from build123d import *

# Parameters (mm, degrees)
SKETCH1_R           = 31.0896
BOSS_EXTRUDE1_DEPTH = 16.002
BOSS_EXTRUDE2_START = -6.35
BOSS_EXTRUDE2_DEPTH = 6.35
FILLET2_R           = 6.35
CUT_EXTRUDE2_REACH  = 96.198
SKETCH4_R           = 1.778
SKETCH4_R_2         = 6.35
SKETCH7_R           = 2.0193
CUT_EXTRUDE4_DEPTH  = 95.197625109
FILLET7_R           = 6.35
FILLET8_R           = 41.148
CUT_EXTRUDE5_DEPTH  = 12.7
FILLET9_R           = 2.54
SKETCH9_R           = 6.35
CUT_EXTRUDE6_DEPTH  = 3.302


# Some blends are built 0.0001 mm under size
with BuildPart() as part:
    # Sketch1 → Boss-Extrude1 (new body)
    with BuildSketch(Plane(origin=(0, 0, 0), x_dir=(1, 0, 0), z_dir=(0, 1, 0))):
        with Locations(Location((0, 0, 0), (0, 0, 270))):
            Circle(SKETCH1_R)
    extrude(amount=BOSS_EXTRUDE1_DEPTH)

    # Sketch2 → Boss-Extrude2 (add)
    with BuildSketch(Plane(origin=(0, 16.002, 0), x_dir=(1, 0, 0), z_dir=(0, 1, 0)).offset(BOSS_EXTRUDE2_START)):
        with BuildLine():
            Line((-31.0896, 0), (-31.0896, 41.148))
            Line((-31.0896, 41.148), (83.2104, 41.148))
            Line((83.2104, 41.148), (83.2104, 15.748))
            Line((83.2104, 15.748), (31.0896, 15.748))
            Line((31.0896, 15.748), (31.0896, 0))
            ThreePointArc((31.0896, 0), (0, -31.0896), (-31.0896, 0))
        make_face()
    extrude(amount=BOSS_EXTRUDE2_DEPTH)

    # Fillet2
    fillet2_edges = [part.edges().sort_by_distance(p)[0] for p in [
        (31.0896, 12.827, -15.748),
    ]]
    fillet(fillet2_edges, radius=FILLET2_R)

    # Sketch4 → Cut-Extrude2 (cut, up to next)
    with BuildSketch(Plane(origin=(0, 16.002, 0), x_dir=(1, 0, 0), z_dir=(0, 1, 0)), mode=Mode.PRIVATE) as cut_extrude2_sk1:
        with Locations(Location((61.411202787, 35.362797213, 0), (0, 0, 270))):
            Circle(SKETCH4_R)
    cut_extrude2_tool1 = extrude(cut_extrude2_sk1.sketch, amount=-CUT_EXTRUDE2_REACH, mode=Mode.PRIVATE) & part.part
    # Sketch4 → Cut-Extrude2 (cut, up to next)
    with BuildSketch(Plane(origin=(0, 16.002, 0), x_dir=(1, 0, 0), z_dir=(0, 1, 0)), mode=Mode.PRIVATE) as cut_extrude2_sk2:
        with Locations(Location((75.240797213, 35.362797213, 0), (0, 0, 270))):
            Circle(SKETCH4_R)
    cut_extrude2_tool2 = extrude(cut_extrude2_sk2.sketch, amount=-CUT_EXTRUDE2_REACH, mode=Mode.PRIVATE) & part.part
    # Sketch4 → Cut-Extrude2 (cut, up to next)
    with BuildSketch(Plane(origin=(0, 16.002, 0), x_dir=(1, 0, 0), z_dir=(0, 1, 0)), mode=Mode.PRIVATE) as cut_extrude2_sk3:
        with Locations(Location((75.240797213, 21.533202787, 0), (0, 0, 270))):
            Circle(SKETCH4_R)
    cut_extrude2_tool3 = extrude(cut_extrude2_sk3.sketch, amount=-CUT_EXTRUDE2_REACH, mode=Mode.PRIVATE) & part.part
    # Sketch4 → Cut-Extrude2 (cut, up to next)
    with BuildSketch(Plane(origin=(0, 16.002, 0), x_dir=(1, 0, 0), z_dir=(0, 1, 0)), mode=Mode.PRIVATE) as cut_extrude2_sk4:
        with Locations(Location((68.326, 28.448, 0), (0, 0, 270))):
            Circle(SKETCH4_R_2)
    cut_extrude2_tool4 = extrude(cut_extrude2_sk4.sketch, amount=-CUT_EXTRUDE2_REACH, mode=Mode.PRIVATE) & part.part
    # Sketch4 → Cut-Extrude2 (cut, up to next)
    with BuildSketch(Plane(origin=(0, 16.002, 0), x_dir=(1, 0, 0), z_dir=(0, 1, 0)), mode=Mode.PRIVATE) as cut_extrude2_sk5:
        with Locations(Location((61.411202787, 21.533202787, 0), (0, 0, 270))):
            Circle(SKETCH4_R)
    cut_extrude2_tool5 = extrude(cut_extrude2_sk5.sketch, amount=-CUT_EXTRUDE2_REACH, mode=Mode.PRIVATE) & part.part
    add(cut_extrude2_tool1.solids().sort_by_distance((61.411203, 16.002, -35.362797))[0], mode=Mode.SUBTRACT)
    add(cut_extrude2_tool2.solids().sort_by_distance((75.240797, 16.002, -35.362797))[0], mode=Mode.SUBTRACT)
    add(cut_extrude2_tool3.solids().sort_by_distance((75.240797, 16.002, -21.533203))[0], mode=Mode.SUBTRACT)
    add(cut_extrude2_tool4.solids().sort_by_distance((68.326, 16.002, -28.448))[0], mode=Mode.SUBTRACT)
    add(cut_extrude2_tool5.solids().sort_by_distance((61.411203, 16.002, -21.533203))[0], mode=Mode.SUBTRACT)

    # Sketch7 → Cut-Extrude4 (cut, through all)
    with BuildSketch(Plane(origin=(0, 0, 0), x_dir=(1, 0, 0), z_dir=(0, 1, 0))):
        with BuildLine():
            ThreePointArc((27.94, 0), (22.235278576, 16.918510179), (7.450666667, 26.928259621))
            Line((7.450666667, 26.928259621), (4.402666667, 15.912153412))
            ThreePointArc((4.402666667, 15.912153412), (13.139028249, 9.997301469), (16.51, 0))
            ThreePointArc((16.51, 0), (13.139028249, -9.997301469), (4.402666667, -15.912153412))
            Line((4.402666667, -15.912153412), (7.450666667, -26.928259621))
            ThreePointArc((7.450666667, -26.928259621), (22.235278576, -16.918510179), (27.94, 0))
        make_face()
        with BuildLine():
            Line((-15.912153412, -4.402666667), (-26.928259621, -7.450666667))
            ThreePointArc((-26.928259621, -7.450666667), (-19.756563466, -19.756563466), (-7.450666667, -26.928259621))
            Line((-7.450666667, -26.928259621), (-4.402666667, -15.912153412))
            ThreePointArc((-4.402666667, -15.912153412), (-11.674332957, -11.674332957), (-15.912153412, -4.402666667))
        make_face()
        with BuildLine():
            Line((-4.402666667, 15.912153412), (-7.450666667, 26.928259621))
            ThreePointArc((-7.450666667, 26.928259621), (-19.756563466, 19.756563466), (-26.928259621, 7.450666667))
            Line((-26.928259621, 7.450666667), (-15.912153412, 4.402666667))
            ThreePointArc((-15.912153412, 4.402666667), (-11.674332957, 11.674332957), (-4.402666667, 15.912153412))
        make_face()
        with Locations(Location((-19.05, 0, 0), (0, 0, 270))):
            Circle(SKETCH7_R)
        with Locations(Location((0, -19.05, 0), (0, 0, 270))):
            Circle(SKETCH7_R)
        with Locations(Location((0, 19.05, 0), (0, 0, 270))):
            Circle(SKETCH7_R)
    extrude(amount=CUT_EXTRUDE4_DEPTH, mode=Mode.SUBTRACT)

    # Fillet7
    # the kernel refuses this fillet: 6.35 mm, written as the material it adds along each edge
    with BuildSketch(Plane(origin=(-26.928259621, 0, -7.450666667), x_dir=(0.40702884348062, 0, -0.9134153056385845), z_dir=(0, 1, 0)), Plane(origin=(-7.450666667, 0, 26.928259621), x_dir=(-0.9134153056385848, 0, -0.40702884348061963), z_dir=(0, 1, 0))) as fillet7_piece_1:
        with BuildLine():
            CenterArc((7.365726845, -6.279391075), FILLET7_R, 81.447682412, 107.104635177)
            Line((1.086335771, -7.223715029), (0, 0))
            ThreePointArc((0, 0), (4.1550254, 0.310679271), (8.3100508, 0))
        make_face()
    extrude(amount=16.002)
    with BuildSketch(Plane(origin=(-7.450666667, 0, -26.928259621), x_dir=(0.26666666666666705, 0, 0.9637888196533972), z_dir=(0, 1, 0)), Plane(origin=(7.450666667, 0, 26.928259621), x_dir=(-0.26666666666666733, 0, -0.9637888196533971), z_dir=(0, 1, 0)), Plane(origin=(-26.928259621, 0, 7.450666667), x_dir=(0.9637888196533975, 0, -0.26666666666666644), z_dir=(0, 1, 0))) as fillet7_piece_2:
        with BuildLine():
            CenterArc((7.304942452, -6.35), FILLET7_R, 90, 107.104635177)
            ThreePointArc((1.235807879, -8.217647059), (0.310679271, -4.1550254), (0, 0))
            Line((0, 0), (7.304942452, 0))
        make_face()
    extrude(amount=16.002)
    with BuildSketch(Plane(origin=(-4.402666667, 0, -15.912153412), x_dir=(-0.916852417954672, 0, 0.39922630636103035), z_dir=(0, 1, 0)), Plane(origin=(4.402666667, 0, 15.912153412), x_dir=(0.9168524179546733, 0, -0.39922630636102746), z_dir=(0, 1, 0)), Plane(origin=(-15.912153412, 0, 4.402666667), x_dir=(0.39922630636102946, 0, 0.9168524179546725), z_dir=(0, 1, 0))) as fillet7_piece_3:
        with BuildLine():
            CenterArc((5.522661099, -6.287214109), FILLET7_R, 98.063810107, 73.872379787)
            Line((-0.76455301, -5.396462319), (0, 0))
            ThreePointArc((0, 0), (2.315954654, -0.163243317), (4.631909309, 0))
        make_face()
    extrude(amount=16.002)
    with BuildSketch(Plane(origin=(4.402666667, 0, -15.912153412), x_dir=(0.26666666666666416, 0, -0.9637888196533979), z_dir=(0, 1, 0))) as fillet7_piece_4:
        with BuildLine():
            CenterArc((5.450352912, -6.35), FILLET7_R, 90, 73.872379787)
            ThreePointArc((-0.649745119, -4.586111111), (-0.163243317, -2.315954654), (0, 0))
            Line((0, 0), (5.450352912, 0))
        make_face()
    extrude(amount=16.002)
    with BuildSketch(Plane(origin=(7.450666667, 0, -26.928259621), x_dir=(-0.2666666666666666, 0, 0.9637888196533974), z_dir=(0, 1, 0))) as fillet7_piece_5:
        with BuildLine():
            CenterArc((7.304942452, 6.35), FILLET7_R, 162.895364823, 107.104635177)
            ThreePointArc((1.235807879, 8.217647059), (0.310679271, 4.1550254), (0, 0))
            Line((0, 0), (7.304942452, 0))
        make_face()
    extrude(amount=16.002)
    with BuildSketch(Plane(origin=(-4.402666667, 0, 15.912153412), x_dir=(-0.9168524179546729, 0, -0.3992263063610288), z_dir=(0, 1, 0)), Plane(origin=(-15.912153412, 0, -4.402666667), x_dir=(0.39922630636102996, 0, -0.9168524179546723), z_dir=(0, 1, 0))) as fillet7_piece_6:
        with BuildLine():
            CenterArc((5.522661099, 6.287214109), FILLET7_R, 188.063810107, 73.872379787)
            Line((-0.76455301, 5.396462319), (0, 0))
            ThreePointArc((0, 0), (2.315954654, 0.163243317), (4.631909309, 0))
        make_face()
    extrude(amount=16.002)

    # Fillet8
    fillet8_edges = [part.edges().sort_by_distance(p)[0] for p in [
        (-31.0896, 12.827, -41.148),
    ]]
    fillet(fillet8_edges, radius=FILLET8_R - 0.0001)  # a hair under: the kernel refuses the full size

    # Sketch8 → Cut-Extrude5 (cut)
    with BuildSketch(Plane.XZ):
        with BuildLine():
            Line((-10.414, 10.414), (10.414, 10.414))
            ThreePointArc((10.414, 10.414), (20.828, 0), (10.414, -10.414))
            Line((10.414, -10.414), (-10.414, -10.414))
            Line((-10.414, -10.414), (-10.414, 10.414))
        make_face()
    extrude(amount=-CUT_EXTRUDE5_DEPTH, mode=Mode.SUBTRACT)

    # Fillet9
    # the kernel refuses this fillet: 2.54 mm, written as the material it takes off along each edge
    with BuildSketch(Plane(origin=(13.087195122, 12.7, 10.065059555), x_dir=(-0.7525451578932851, 0, 0.658540648199768), z_dir=(0, -1, 0))) as fillet9_piece_1:
        with BuildLine():
            CenterArc((7.288242174, 2.538935053), FILLET9_R, 131.188669075, 137.152126286)
            Line((5.615548928, 4.450399754), (5.448279603, 4.641546224))
            ThreePointArc((5.448279603, 4.641546224), (2.074222188, 1.688960676), (-0.1125988, 0.227678524))
            Line((-0.1125988, 0.227678524), (-0.049545453, -0.249120951))
            ThreePointArc((-0.049545453, -0.249120951), (6.014734512, -0.336617786), (7.207343199, -0.253893505))
            Line((7.207343199, -0.253893505), (7.214697651, 0))
        make_face()
    extrude(amount=30.736744128, mode=Mode.SUBTRACT)
    with BuildSketch(Plane(origin=(13.087195122, 12.7, -10.065059555), x_dir=(-0.7525451578933744, 0, -0.658540648199666), z_dir=(0, -1, 0))) as fillet9_piece_2:
        with BuildLine():
            CenterArc((7.288242174, -2.538935053), FILLET9_R, 91.659204639, 137.152126286)
            Line((5.615548928, -4.450399754), (5.448279603, -4.641546224))
            ThreePointArc((5.448279603, -4.641546224), (2.074222188, -1.688960676), (-0.1125988, -0.227678524))
            Line((-0.1125988, -0.227678524), (-0.049545453, 0.249120951))
            ThreePointArc((-0.049545453, 0.249120951), (6.014734512, 0.336617786), (7.207343199, 0.253893505))
            Line((7.207343199, 0.253893505), (7.214697651, 0))
        make_face()
    extrude(amount=30.736744128, mode=Mode.SUBTRACT)

    # Sketch9 → Cut-Extrude6 (cut)
    with BuildSketch(Plane.XZ.offset(-12.7)):
        with Locations(Location((0, 0, 0), (0, 0, 270))):
            Circle(SKETCH9_R)
    extrude(amount=-CUT_EXTRUDE6_DEPTH, mode=Mode.SUBTRACT)


solid = part.part
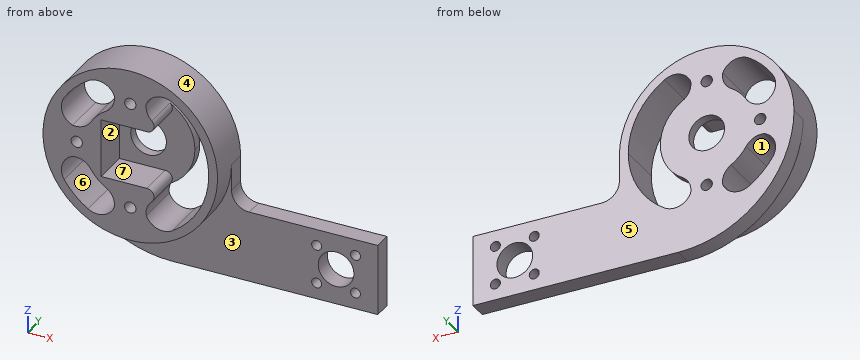
For this review, take the finished solid that the model builds, in its own axes (mm). Face numbers are marked on the shaded views. A direction names the side the tool comes from. Round coordinates to 2 decimals unless told otherwise and drop trailing zeros. Order: outer loops, then holes, each group sorted by start corner. A loop starts at its lowest first (then second) coordinate and runs counter-clockwise, first axis right, second up. Notation, with made-up numbers: M 0,19 L 23,19 A32 cw 23,47 Z; hole C -12.75,15 d9. An arc over 180 degrees is marked long. Use a Markdown table: item, result. Add a question column.
Item 1: Add section A-A, the plane x = 20.5. Give the boundary of the cut face in (y, z).
Item 2: Add section C-C, the plane z = 19.05. Give the boundary of the cut face in (x, y), then the cut area to 3 significant figures.
Item 3: Add section B-B, the plane x = -19.05. Give the boundary of the cut face in (y, z).
Item 4: Tool access review of the marked faces 5, 6 and 7: name each direction out of +Z, -Z, +X, -X, +Y, -Y from which nothing blocks a thin tool from reaching the whole face with its end or side.
Item 5: Mouldability with a two-part tool opening along Z and no side actions: class the marked faces 1, 2, 3 and 4 as released by +Z, released by -Z, zero draft, split by the parting line, or undercut.
Item 6: Add section D-D, the plane y = 1.5. Give the boundary of the cut face in (x, z).
Item 7: To check wall thickness, follow line 1 along X through (y, z) = (14, -7); line 2 along X through (y, z) = (12, 9.5); line 3 along X through (y, z) = (14, -31.5). State the ranges of each line that lie inside material, in increasing order.
Item 8: Insertion check: pin 1 (4 mm diameter, centred on x = 75.24, z = -35.36, fed in from -Y); pin 2 (1.5 mm diameter, centred on y = 7, z = 6.5, fed in from -X); pin 3 (4 mm diameter, centred on y = 3, z = -15, fed in from -X). Each pin has a flat end and moves straight along its axis. Give the tip position at first contact, or say it passes through.
Geometry results:
| question | item | result |
|---|---|---|
| 1 | outline | M 0,-23.37 L 9.65,-23.37 L 9.65,-41.15 L 16,-41.15 L 16,-18.98 L 0,-18.98 Z; M 0,18.98 L 16,18.98 L 16,23.37 L 0,23.37 Z |
| 2 | outline | M -24.57,0 L -20.44,0 L -20.44,16 L -24.57,16 Z; M -5.64,0 L -2.02,0 L -2.02,16 L -5.64,16 Z; M 2.02,0 L 5.64,0 L 5.64,16 L 2.02,16 Z; M 20.44,0 L 24.57,0 L 24.57,16 L 20.44,16 Z |
| 2 | area | 248 mm² |
| 3 | outline | M 0,-24.57 L 9.65,-24.57 L 9.65,-29.08 L 16,-29.08 L 16,-20.44 L 0,-20.44 Z; M 0,-5.64 L 16,-5.64 L 16,-2.02 L 0,-2.02 Z; M 0,2.02 L 16,2.02 L 16,5.64 L 0,5.64 Z; M 0,20.44 L 16,20.44 L 16,24.57 L 0,24.57 Z |
| 4 | face 5 | +Z, -Z, +X, -X, +Y |
| 4 | face 6 | +Y, -Y |
| 4 | face 7 | -Y |
| 5 | face 1 | undercut |
| 5 | face 2 | undercut |
| 5 | face 3 | zero draft |
| 5 | face 4 | split by the parting line |
| 6 | outline | C 0,0 d62.18; hole M -23.55,-15.04 A27.94 ccw -15.04,-23.55 A6.35 ccw -5.71,-20.52 A6.35 ccw -8.65,-14.06 A16.51 cw -14.06,-8.65 A6.35 ccw -20.52,-5.71 A6.35 ccw Z; hole M -23.55,15.04 A6.35 ccw -20.52,5.71 A6.35 ccw -14.06,8.65 A16.51 cw -8.65,14.06 A6.35 ccw -5.71,20.52 A6.35 ccw -15.04,23.55 A27.94 ccw Z; hole C -19.05,0 d4.04; hole M -10.41,-10.41 L 5.93,-10.41 A2.54 cw 7.66,-14.82 A6.35 ccw 5.71,-20.52 A6.35 ccw 15.04,-23.55 A27.94 ccw 15.04,23.55 A6.35 ccw 5.71,20.52 A6.35 ccw 7.66,14.82 A2.54 cw 5.93,10.41 L -10.41,10.41 Z; hole C 0,-19.05 d4.04; hole C 0,19.05 d4.04 |
| 7 | line 1 | x = -30.49 to -22.55, -15.53 to 14.95, 27.05 to 31.09 |
| 7 | line 2 | x = -29.6 to -24.18, -13.5 to -10.41, 26.28 to 29.6 |
| 7 | line 3 | x = -16.42 to 62.76, 73.89 to 83.21 |
| 8 | pin 1 | stops at y = 9.65 |
| 8 | pin 2 | stops at x = -30.55 |
| 8 | pin 3 | stops at x = -28.24 |
